from build123d import *

# Parameters (mm, degrees)
F0_W     = 44.8
F0_H     = 16
F1_DEPTH = 2
F4_DEPTH = 5
F5_DEPTH = 5
F6_W     = 2
F6_H     = 16
F7_DEPTH = 7


# Not quite as in the source:
# - a pattern or mirror of a feature is missing from the dataset's text; its kind, count and spacing are read off the source's solid


with BuildPart() as f1:
    # F0 (on Top) → F1 (new body)
    with BuildSketch(Plane.XY):
        Rectangle(F0_W, F0_H)
    extrude(amount=F1_DEPTH)

    # F2 (on face) → F4 (join)
    with BuildSketch(Plane.XY.offset(2)):
        with BuildLine():
            Line((-19.9, 3.6), (-19.9, -8))
            Line((-19.9, -8), (-18.9, -8))
            Line((-18.9, -8), (-18.9, 3.6))
            ThreePointArc((-18.9, 3.6), (-18.6071067812, 4.3071067812), (-17.9, 4.6))
            Line((-17.9, 4.6), (-9.4, 4.6))
            ThreePointArc((-9.4, 4.6), (-8.6928932188, 4.3071067812), (-8.4, 3.6))
            Line((-8.4, 3.6), (-8.4, -8))
            Line((-8.4, -8), (-7.4, -8))
            Line((-7.4, -8), (-7.4, 3.6))
            ThreePointArc((-7.4, 3.6), (-7.9857864376, 5.0142135624), (-9.4, 5.6))
            Line((-9.4, 5.6), (-17.9, 5.6))
            ThreePointArc((-17.9, 5.6), (-19.3142135624, 5.0142135624), (-19.9, 3.6))
        make_face()
    f4 = extrude(amount=F4_DEPTH)

    # F4_copies: F4 across plane
    add(f4.mirror(Plane(origin=(0, 0, 0), x_dir=(0, 0, 1), z_dir=(1, 0, 0))))

    # F3 (on face) → F5 (join)
    with BuildSketch(Plane.XY.offset(2)):
        with BuildLine():
            Line((4.75, -8), (4.75, -2.45))
            ThreePointArc((4.75, -2.45), (0, 2.3), (-4.75, -2.45))
            Line((-4.75, -2.45), (-4.75, -8))
            Line((-4.75, -8), (4.75, -8))
        make_face()
    extrude(amount=F5_DEPTH)

    # F6 (on Top) → F7 (join, through all)
    with BuildSketch(Plane.XY):
        with Locations((-23.4, 0)):
            Rectangle(F6_W, F6_H)
    f7 = extrude(amount=F7_DEPTH)

    # F7_copies: F7 across plane
    add(f7.mirror(Plane(origin=(0, 0, 0), x_dir=(0, 0, 1), z_dir=(1, 0, 0))))


solid = f1.part
Geometry: final body of the model. Coordinates: model frame, mm. A direction names the side the tool comes from. Round coordinates to 2 decimals unless told otherwise and drop trailing zeros. Loops run counter-clockwise (first coordinate to the right, second up) from the corner with the lowest first, then second, coordinate; pieces in that order, holes last. Notation, with made-up numbers: M 9.25,28 L 37.25,28 A15 ccw 37.25,37 Z; hole C -23.75,64.5 d1. An arc over 180 degrees is marked long. Put each result on its own line as item: value. Start each with the question number.
(1) Material intervals for line 1 along X through (y, z) = (2.5, 6); line 2 along X through (y, z) = (6.5, 5.25); line 3 along X through (y, z) = (5, 3.25), sorted ascending. Write a range as [from, to].
(2) Contact query for flat-ended pins moving along their axis: pin 1 Ø2.5 at (x, z) = (12, 5) entering from -Y; pin 2 Ø3 at (x, y) = (14.5, -0.5) entering from +Z. Output: stop coordinate, or through.
(3) Draft query along X for faces 5 (the face through (-24.4, 0, 3)), 6 (the face through (19.3, 5.03, 4.46)), 7 (the face through (-23, 0, 7)). Return one class per face: +X half, -X half, draft (parallel to the pull), parting line (faces both ways), or undercut.
(4) Section query D-D (x = -12). Return loops of the section in (y, z), then the cut area to 3 significant figures.
(5) Set-up query: faces 1 (the face through (18.9, -2, 4)), 2 (the face through (0, -8, 2)), 3 (the face through (4.75, -5, 4)), 4 (the face through (-19.3, 5.03, 4.46)). Return all of +Z, -Z, +X, -X, +Y, -Y with unobstructed straight access to the full face (end or side cutting, diameter ignored); none if empty.
(6) Section query A-A (y = -4.75). Return loops of the section in (x, z).
(7) Section query B-B (x = 0). Return loops of the section in (y, z).
(8) Section query C-C (z = 2.5). State how many separate pieces and enclosed holes the cut face has, then the cut area to 3 significant figures.
Findings below:
1. line 1: x = [-24.4, -22.4], [-19.9, -18.9], [-8.4, -7.4], [7.4, 8.4], [18.9, 19.9], [22.4, 24.4]
1. line 2: x = [-24.4, -22.4], [22.4, 24.4]
1. line 3: x = [-24.4, -22.4], [-19.33, -7.97], [7.97, 19.33], [22.4, 24.4]
2. pin 1: stops at y = 4.6
2. pin 2: stops at z = 2
3. face 5: -X half
3. face 6: undercut
3. face 7: draft
4. outline: M -8,0 L 8,0 L 8,2 L 5.6,2 L 5.6,7 L 4.6,7 L 4.6,2 L -8,2 Z
4. area: 37.0 mm2
5. face 1: +Z, -Y
5. face 2: +Z, -Z, +X, -X, -Y
5. face 3: +Z, +Y, -Y
5. face 4: +Z, +Y
6. outline: M -24.4,0 L 24.4,0 L 24.4,7 L 22.4,7 L 22.4,2 L 19.9,2 L 19.9,7 L 18.9,7 L 18.9,2 L 8.4,2 L 8.4,7 L 7.4,7 L 7.4,2 L 4.75,2 L 4.75,7 L -4.75,7 L -4.75,2 L -7.4,2 L -7.4,7 L -8.4,7 L -8.4,2 L -18.9,2 L -18.9,7 L -19.9,7 L -19.9,2 L -22.4,2 L -22.4,7 L -24.4,7 Z
7. outline: M -8,0 L 8,0 L 8,2 L 2.3,2 L 2.3,7 L -8,7 Z
8. separate pieces: 5
8. enclosed holes: 0
8. area: 225 mm2
